Geometry: final body of the model. Coordinates: model frame, mm. A direction names the side the tool comes from. Coordinates: 2 decimals unless noted, no trailing zeros. Order: outer loops, then holes, each group sorted by start corner. A loop starts at its lowest first (then second) coordinate and runs counter-clockwise, first axis right, second up. Notation, with made-up numbers: (49, 60) - (107, 60) arc R13 cw to (107, 78) - close; hole circle Ø6 at (-27.5, 15.25). An arc over 180 degrees is marked (long way). Use a Markdown table: item, result. Add a question column.
```python
from build123d import *

# Parameters (mm, degrees)
SKETCH1_W                           = 184.15
SKETCH1_H                           = 39.6875
EXTRUDE1_DEPTH                      = 34.925
SKETCH2_W                           = 31.75
SKETCH2_H                           = 44.45
EXTRUDE2_DEPTH                      = 69.85
EXTRUDE3_DEPTH                      = 25.4
CUT_EXTRUDE1_START                  = -15.24
CUT_EXTRUDE1_DEPTH                  = 169.91
EXTRUDE4_DEPTH                      = 7.9375
EXTRUDE5_DEPTH                      = 7.9375
SKETCH17_W                          = 82.55
SKETCH17_H                          = 12.7
EXTRUDE7_DEPTH                      = 7.9375
F_1_2_0_5_DIAMETER_HOLE1_D          = 12.7
EXTRUDE6_DEPTH                      = 27.94
F_1_4_0_25_DIAMETER_HOLE2_D         = 6.35
F_1_4_0_25_DIAMETER_HOLE2_DEPTH     = 15.875
F_1_4_0_25_DIAMETER_HOLE2_TIP       = 1.907732465
F_11_16_0_6875_DIAMETER_HOLE1_D     = 17.4625
F_11_16_0_6875_DIAMETER_HOLE1_DEPTH = 25.4
FILLET15_R                          = 3.175


with BuildPart() as part:
    # Sketch1 → Extrude1 (new body, symmetric)
    with BuildSketch(Plane.XY):
        with Locations((92.075, 19.84375)):
            Rectangle(SKETCH1_W, SKETCH1_H)
    extrude(amount=EXTRUDE1_DEPTH, both=True)

    # Sketch2 → Extrude2 (add)
    with BuildSketch(Plane.XY.offset(34.925)):
        with Locations((15.875, 61.9125)):
            Rectangle(SKETCH2_W, SKETCH2_H)
    extrude(amount=-EXTRUDE2_DEPTH)

    # Sketch3 → Extrude3 (add)
    with BuildSketch(Plane(origin=(184.15, 0, 0), x_dir=(0, 0, -1), z_dir=(1, 0, 0))):
        with BuildLine():
            Line((-34.925, 39.6875), (34.925, 39.6875))
            Line((34.925, 39.6875), (34.925, 55.929117421))
            Line((34.925, 55.929117421), (8.89, 70.960431679))
            ThreePointArc((8.89, 70.960431679), (0, 73.3425), (-8.89, 70.960431679))
            Line((-8.89, 70.960431679), (-34.925, 55.929117421))
            Line((-34.925, 55.929117421), (-34.925, 39.6875))
        make_face()
    extrude(amount=-EXTRUDE3_DEPTH)

    # Sketch4 → Cut-Extrude1 (cut, through all)
    with BuildSketch(Plane(origin=(184.15, 0, 0), x_dir=(0, 0, -1), z_dir=(1, 0, 0)).offset(CUT_EXTRUDE1_START)):
        Polygon((-15.875, 0), (15.875, 0), (15.875, 26.9875), (12.7, 26.9875), (12.7, 42.8625), (-12.7, 42.8625), (-12.7, 26.9875), (-15.875, 26.9875), align=None)
    extrude(amount=-CUT_EXTRUDE1_DEPTH, mode=Mode.SUBTRACT)

    # Sketch5 → Extrude4 (add)
    with BuildSketch(Plane.XZ):
        with BuildLine():
            Line((50.8, 53.975), (50.8, 34.925))
            Line((50.8, 34.925), (0, 34.925))
            Line((0, 34.925), (0, 53.975))
            ThreePointArc((0, 53.975), (25.4, 79.375), (50.8, 53.975))
        make_face()
    extrude4 = extrude(amount=-EXTRUDE4_DEPTH)

    # Sketch6 → Extrude5 (add)
    with BuildSketch(Plane.XZ):
        with BuildLine():
            Line((184.15, 34.925), (133.35, 34.925))
            Line((133.35, 34.925), (133.35, 53.975))
            ThreePointArc((133.35, 53.975), (158.75, 79.375), (184.15, 53.975))
            Line((184.15, 53.975), (184.15, 34.925))
        make_face()
    extrude5 = extrude(amount=-EXTRUDE5_DEPTH)

    # Sketch17 → Extrude7 (add)
    with BuildSketch(Plane.XZ):
        with Locations((92.075, 41.275)):
            Rectangle(SKETCH17_W, SKETCH17_H)
    extrude7 = extrude(amount=-EXTRUDE7_DEPTH)

    # 1/2 (0.5) Diameter Hole1 (through all)
    with Locations(Plane(origin=(0, 7.9375, 0), x_dir=(-1, 0, 0), z_dir=(0, 1, 0))):
        with Locations((-25.4, 53.975), (-158.75, 53.975)):
            f_1_2_0_5_diameter_hole1 = Hole(F_1_2_0_5_DIAMETER_HOLE1_D / 2)

    # Mirror1: Extrude4, Extrude5, Extrude7, 1/2 (0.5) Diameter Hole1 across plane
    add(extrude4.mirror(Plane.XY))
    add(extrude5.mirror(Plane.XY))
    add(extrude7.mirror(Plane.XY))
    add(f_1_2_0_5_diameter_hole1.mirror(Plane.XY), mode=Mode.SUBTRACT)

    # Sketch16 → Extrude6 (add)
    with BuildSketch(Plane(origin=(0, 0, 0), x_dir=(0, 0, -1), z_dir=(1, 0, 0))):
        with BuildLine():
            Line((-34.925, 84.1375), (34.925, 84.1375))
            Line((34.925, 84.1375), (34.925, 84.504117421))
            Line((34.925, 84.504117421), (8.89, 99.535431679))
            ThreePointArc((8.89, 99.535431679), (0, 101.9175), (-8.89, 99.535431679))
            Line((-8.89, 99.535431679), (-34.925, 84.504117421))
            Line((-34.925, 84.504117421), (-34.925, 84.1375))
        make_face()
    extrude(amount=EXTRUDE6_DEPTH)

    # 1/4 (0.25) Diameter Hole2
    with Locations(Plane(origin=(31.75, 0, 0), x_dir=(0, 0, -1), z_dir=(1, 0, 0))):
        with Locations((-19.05, 65.0875), (19.05, 65.0875)):
            Hole(F_1_4_0_25_DIAMETER_HOLE2_D / 2, depth=F_1_4_0_25_DIAMETER_HOLE2_DEPTH)
            with Locations((0, 0, -(F_1_4_0_25_DIAMETER_HOLE2_DEPTH + F_1_4_0_25_DIAMETER_HOLE2_TIP / 2))):  # 118° drill point
                Cone(0, F_1_4_0_25_DIAMETER_HOLE2_D / 2, F_1_4_0_25_DIAMETER_HOLE2_TIP, mode=Mode.SUBTRACT)

    # 11/16 (0.6875) Diameter Hole1
    with Locations(Plane(origin=(184.15, 0, 0), x_dir=(0, 0, -1), z_dir=(1, 0, 0))):
        with Locations((0, 55.5625)):
            Hole(F_11_16_0_6875_DIAMETER_HOLE1_D / 2, depth=F_11_16_0_6875_DIAMETER_HOLE1_DEPTH)

    # Fillet15
    fillet15_edges = [part.edges().sort_by_distance(p)[0] for p in [
        (158.75, 47.80830871, 34.925),
        (158.75, 47.80830871, -34.925),
    ]]
    fillet(fillet15_edges, radius=FILLET15_R)


solid = part.part
```
1) Section query C-C (y = 30). Return the cut outline in (x, z) (3 decimals), and give its area (3 significant figures).
2) Section query B-B (z = 0). Return the cut outline in (x, y), and give its area (3 significant figures).
3) Section query A-A (x = 70). Return the cut outline in (y, z) (1 decimal).
4) Section query D-D (x = 25.4). Give the number of separate pieces and of enclosed holes in the cut face, and give its area (3 significant figures).
5) Line query: line 1 (Z direction, x = 158, y = 4) (3 decimals); line 2 (Z direction, x = 125, y = 26) (3 decimals); line 3 (Z direction, x = 25.4, y = 4.25) (3 decimals). Output: solid intervals per line, ascending. Write a range as from..to.
6) Draft query along X for faces 1 (the flat face through (0, 52, 1)), 2 (the cylindrical face through (24.84, 3.91, 79.37)), 3 (the flat face through (171.63, 63.34, -22.09)). Return one class per face: released by +X, released by -X, zero draft, split by the parting line, or undercut.
7) Access query for faces 4 (the flat face through (91, 4, -47.625)), 5 (the flat face through (31.75, 62, 0)), 6 (the flat face through (91, 7.938, 43)). Directions: +Z, -Z, +X, -X, +Y, -Y. A direction counts if a zero-diameter tool reaches every point of the face in a straight line with its end or side. Return the directions, or none.
8) First-contact query: pin 1 (5 mm diameter, centred on x = 109, y = 34.5, fed in from +Z) (3 decimals); pin 2 (3 mm diameter, centred on x = 80.5, y = 14, fed in from -Z) (3 decimals); pin 3 (4 mm diameter, centred on x = 157.5, z = -20.5, fed in from +Y). Flat tips, straight axial feed; report the tip coordinate or a pass-through.
From the geometry:
| question | item | result |
|---|---|---|
| 1 | outline | (0, -34.925) - (184.15, -34.925) - (184.15, 34.925) - (0, 34.925) - (0, 12.7) - (168.91, 12.7) - (168.91, -12.7) - (0, -12.7) - close |
| 1 | area | 8,570 mm^2 |
| 2 | outline | (0, 42.86) - (31.75, 42.86) - (31.75, 84.14) - (27.94, 84.14) - (27.94, 101.92) - (0, 101.92) - close; (158.75, 42.86) - (168.91, 42.86) - (168.91, 0) - (184.15, 0) - (184.15, 46.83) - (158.75, 46.83) - close; (158.75, 64.29) - (184.15, 64.29) - (184.15, 73.34) - (158.75, 73.34) - close |
| 2 | area | 2,790 mm^2 |
| 3 | outline | (0, -47.6) - (7.9, -47.6) - (7.9, -34.9) - (39.7, -34.9) - (39.7, -12.7) - (27, -12.7) - (27, -15.9) - (0, -15.9) - close; (0, 15.9) - (27, 15.9) - (27, 12.7) - (39.7, 12.7) - (39.7, 34.9) - (7.9, 34.9) - (7.9, 47.6) - (0, 47.6) - close |
| 4 | separate pieces | 3 |
| 4 | enclosed holes | 2 |
| 4 | area | 5,770 mm^2 |
| 5 | line 1 | z = -79.364..-60.281, -47.669..-15.875, 15.875..47.669, 60.281..79.364 |
| 5 | line 2 | z = -34.925..-15.875, 15.875..34.925 |
| 5 | line 3 | z = -79.375..-60.325, -47.625..-15.875, 15.875..47.625, 60.325..79.375 |
| 6 | face 1 | released by -X |
| 6 | face 2 | undercut |
| 6 | face 3 | zero draft |
| 7 | face 4 | -Z, +Y, -Y |
| 7 | face 5 | +Z, -Z, +Y |
| 7 | face 6 | +Z, +X, -X, +Y |
| 8 | pin 1 | stops at z = 34.925 |
| 8 | pin 2 | stops at z = -34.925 |
| 8 | pin 3 | stops at y = 65.16 |
